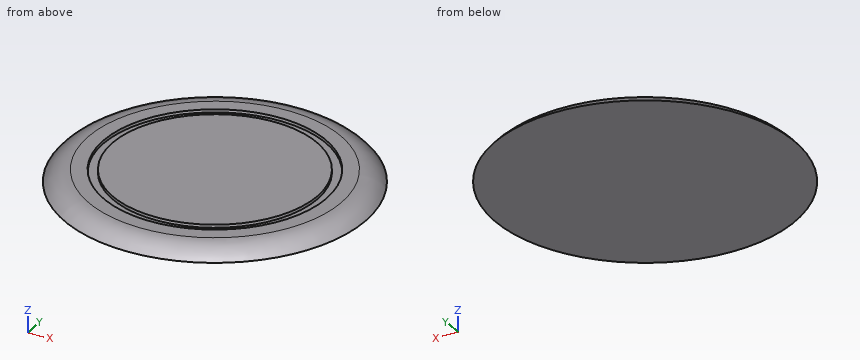
```python
from build123d import *

# Parameters (mm, degrees)
F0_R     = 50
F1_DEPTH = 4
F3_R     = 37
F3_R_2   = 34
F4_DEPTH = 1


# Not quite as in the source:
# - a fillet or chamfer that OpenCascade refuses, or shapes differently, is made with other operations: its cross-section is extruded or revolved along the edge and cut away or added


with BuildPart() as f1:
    # F0 (on Top) → F1 (new body)
    with BuildSketch(Plane.XY):
        Circle(F0_R)
    extrude(amount=F1_DEPTH)

    # F2: fillet of radius 10 on 1 edges, made by hand

    # F2_s1 → F2_t2 (revolve, cut)
    with BuildSketch(Plane.XZ):
        with BuildLine():
            ThreePointArc((50, 0), (46.472135955, 2.94427191), (42, 4))
            Line((42, 4), (50, 4))
            Line((50, 4), (50, 0))
        make_face()
    revolve(axis=Axis((0, 0, 4), (0, 0, 1)), mode=Mode.SUBTRACT)

    # F3 (on face) → F4 (cut)
    with BuildSketch(Plane.XY.offset(4)):
        Circle(F3_R)
        Circle(F3_R_2, mode=Mode.SUBTRACT)
    extrude(amount=-F4_DEPTH, mode=Mode.SUBTRACT)


solid = f1.part
```
Read the model definition and answer for the solid it produces. Units are mm, in the model's axes. Round coordinates to 2 decimals unless told otherwise and drop trailing zeros. Write each loop counter-clockwise with the first axis right and the second up, starting at its lowest first coordinate (ties: lowest second). Pieces come first, ordered by that corner, then holes. Notation, with made-up numbers: (75, 16.25) -> (123, 16.25) arc R34 ccw to (123, 51.25) -> close; hole circle Ø5 at (83, 48). An arc over 180 degrees is marked (long way). Answer in a Markdown table with one row per item. Add a question column.
1) Given P1, Ø4, axis at x = 34.5, y = 36, coming from the -Z side; P2, Ø1.5, axis at x = -24, z = 1.5, coming from the +Y side; P3, Ø1, axis at x = -19.5, z = 3, coming from the -Y side, each flat-ended and moving along its own axis, determine where each tip first touches the part or whether it passes through.
2) Find section C-C, the plane z = 1.8. Determine the outline of the cut face in (x, y).
3) Consider line 1 (X direction, y = 22.5, z = 3.1); line 2 (Y direction, x = -45, z = 0.25); line 3 (X direction, y = -12, z = 1.55). Determine where each line is inside the solid, lowest interval first.
4) Find section A-A, the plane y = 0. Determine the outline of the cut face in (x, z), and give its area (3 significant figures).
Findings below:
| question | item | result |
|---|---|---|
| 1 | P1 | z = 0 |
| 1 | P2 | y = 43.25 |
| 1 | P3 | y = -43.09 |
| 2 | outline | circle Ø96.52 at (0, 0) |
| 3 | line 1 | -40.29 to -29.37, -25.49 to 25.49, 29.37 to 40.29 |
| 3 | line 2 | -21.35 to 21.35 |
| 3 | line 3 | -47.05 to 47.05 |
| 4 | outline | (-50, 0) -> (50, 0) arc R10 ccw to (42, 4) -> (37, 4) -> (37, 3) -> (34, 3) -> (34, 4) -> (-34, 4) -> (-34, 3) -> (-37, 3) -> (-37, 4) -> (-42, 4) arc R10 ccw to start |
| 4 | area | 375 mm² |
